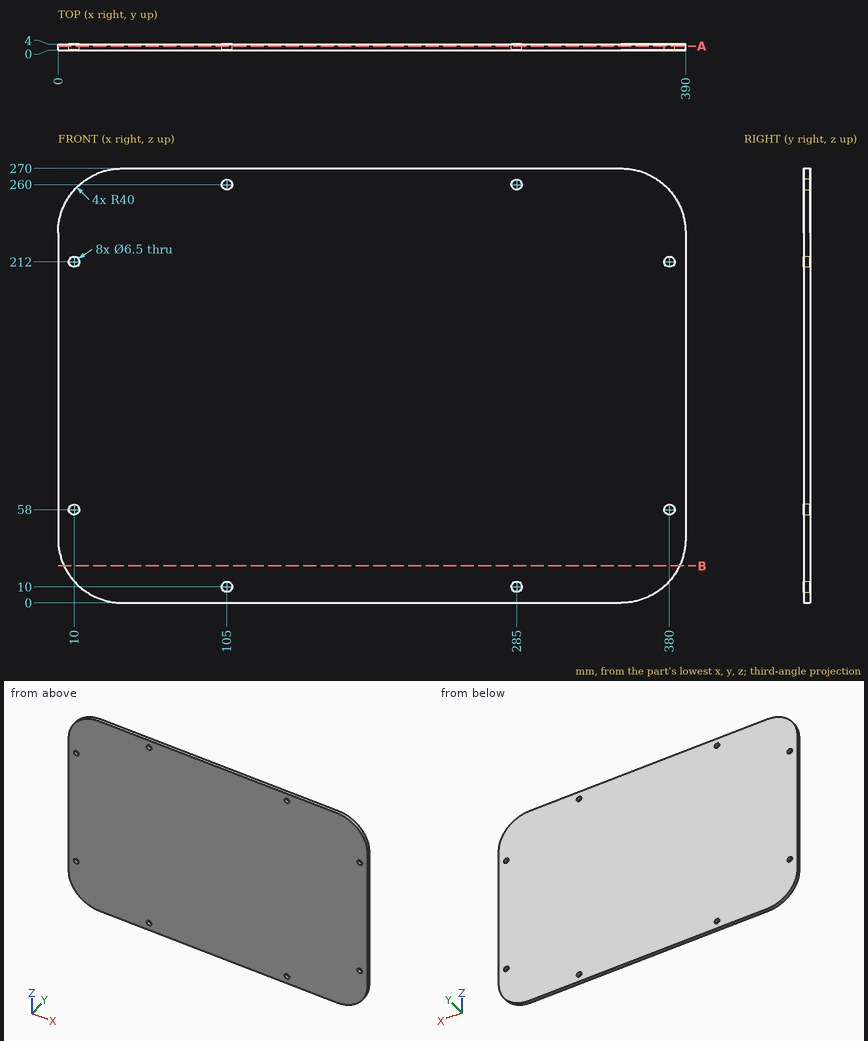
Design review of the part shown in the three views and the two pictorial views. Dimensions are in mm from the part's minimum x, y and z. Round coordinates to 2 decimals unless told otherwise and drop trailing zeros. Loops run counter-clockwise (first coordinate to the right, second up) from the corner with the lowest first, then second, coordinate; pieces in that order, holes last.
Q1. To check wall thickness, follow line 1 along X through (y, z) = (1.65, 58); line 2 along Z through (x, y) = (285, 1.15); line 3 along X through (y, z) = (1.05, 260). State the ranges of each line that lie inside material, in increasing order.
Result sheet:
line 1: x = 0 to 6.75, 13.25 to 376.75, 383.25 to 390
line 2: z = 0 to 6.75, 13.25 to 256.75, 263.25 to 270
line 3: x = 13.54 to 101.75, 108.25 to 281.75, 288.25 to 376.46
Q2. Add section B-B on z = 23. Write out the cut boundary in (x, y).
Result sheet:
outline: (3.79, 0) - (386.21, 0) - (386.21, 4) - (3.79, 4) - close
Q3. Add section A-A on y = 2.6. Give the number of separate pieces and of enclosed holes in the cut face, plus the area to 3 significant figures.
Result sheet:
separate pieces: 1
enclosed holes: 8
area: 104,000 mm2
